Geometry check sheet. Reference: the model listing, model coordinates, mm. Face numbers are marked on the shaded views. A direction names the side the tool comes from. Round coordinates to 2 decimals unless told otherwise and drop trailing zeros. Order: outer loops, then holes, each group sorted by start corner. A loop starts at its lowest first (then second) coordinate and runs counter-clockwise, first axis right, second up. Notation, with made-up numbers: (31.5, -25) - (38.5, -25) arc R6 cw to (38.5, -20) - close; hole circle Ø1 at (27.5, 33.25). An arc over 180 degrees is marked (long way). Use a Markdown table: item, result. Add a question column.
(1) Section check B-B on y = 1.25. Record the boundary of the cut face in (x, z).
(2) Gauge pin test, flat ends, axial feed: P1, Ø1.5, axis at x = 2.5, z = 8, coming from the -Y side; P2, Ø5, axis at x = 0.5, z = 13, coming from the -Y side; P3, Ø2, axis at y = -1, z = 11, coming from the -X side; P4, Ø2, axis at y = 2, z = 6.5, coming from the -X side. Record the tip position at first contact, or that the pin passes through.
(3) Section check D-D on z = 3.5. Record the boundary of the cut face in (x, y).
(4) Mould release check, pull along Y, two halves, no side actions. Record for the marked faces 4, 5 and 6: released by +Y, released by -Y, zero draft, split by the parting line, or undercut.
(5) Section check C-C on x = 4. Record the boundary of the cut face in (y, z), then the cut area to 3 significant figures.
(6) Thickness scan on line 1 along Z through (x, y) = (-1.25, -0.5); line 2 along X through (y, z) = (-1.25, 18); line 3 along Z through (x, y) = (1.5, 3.25). Record the ranges inside material, lowest first. Write a range as [from, to].
(7) Access from +Z, -Z, +X, -X, +Y, -Y to the whole of each face (thin tool, end or side, straight path). Record for the marked faces 1, 2 and 3.
(8) Section check A-A on z = 17.25. Record the boundary of the cut face in (x, y).
```python
from build123d import *

# Parameters (mm, degrees)
SKETCH_1_R           = 3
EXTRUDE_1_DEPTH      = 15
EXTRUDE_2_DEPTH      = 5
EXTRUDE_2_DEPTH_BACK = 1
SKETCH_2_R           = 5


with BuildPart() as part:
    # 草图1 → 拉伸1 (new body)
    with BuildSketch(Plane.XY):
        Circle(SKETCH_1_R)
    extrude(amount=EXTRUDE_1_DEPTH)

    # 草图2 → 拉伸2 (add, two sides: drawn at the far end of the back side and taken through both)
    with BuildSketch(Plane.XY.offset(15).offset(-EXTRUDE_2_DEPTH_BACK)):
        Circle(SKETCH_2_R)
        Polygon((-1.830187787, 2.305076164), (-2.911348409, -0.432451036), (-1.081160622, -2.7375272), (1.830187787, -2.305076164), (2.911348409, 0.432451036), (1.081160622, 2.7375272), align=None, mode=Mode.SUBTRACT)
    extrude(amount=EXTRUDE_2_DEPTH + EXTRUDE_2_DEPTH_BACK)


solid = part.part
```
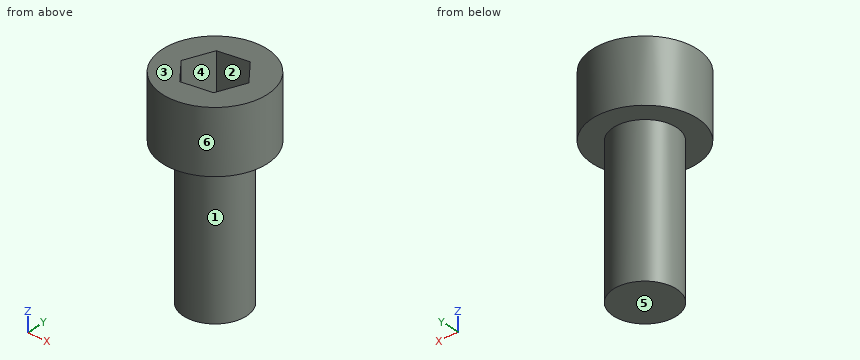
Check sheet entries:
| question | item | result |
|---|---|---|
| 1 | outline | (-4.84, 14) - (-2.73, 14) - (-2.73, 0) - (2.73, 0) - (2.73, 14) - (4.84, 14) - (4.84, 20) - (2.26, 20) - (2.26, 15) - (-2.25, 15) - (-2.25, 20) - (-4.84, 20) - close |
| 2 | P1 | stops at y = -2.44 |
| 2 | P2 | stops at y = -5 |
| 2 | P3 | stops at x = -3 |
| 2 | P4 | stops at x = -2.83 |
| 3 | outline | circle Ø6 at (0, 0) |
| 4 | face 4 | undercut |
| 4 | face 5 | zero draft |
| 4 | face 6 | split by the parting line |
| 5 | outline | (-3, 14) - (3, 14) - (3, 20) - (-3, 20) - close |
| 5 | area | 36.0 mm2 |
| 6 | line 1 | z = [0, 15] |
| 6 | line 2 | x = [-4.84, -2.26], [2.25, 4.84] |
| 6 | line 3 | z = [14, 20] |
| 7 | face 1 | -Z |
| 7 | face 2 | +Z |
| 7 | face 3 | +Z, +X, -X, +Y, -Y |
| 8 | outline | circle Ø10 at (0, 0); hole (-2.91, -0.43) - (-1.08, -2.74) - (1.83, -2.31) - (2.91, 0.43) - (1.08, 2.74) - (-1.83, 2.31) - close |
